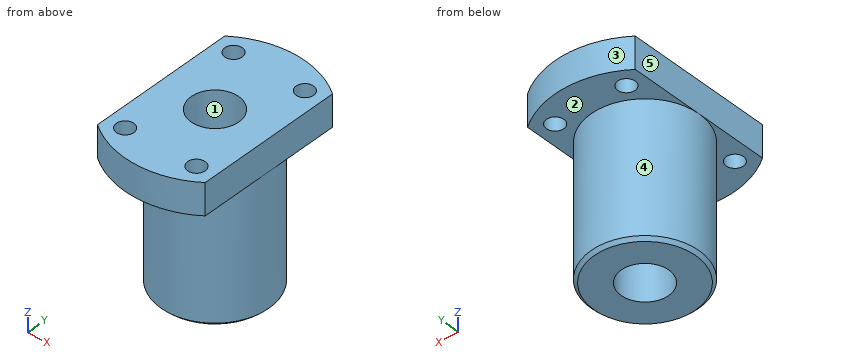
```python
from build123d import *

# Parameters (mm, degrees)
SKETCH_1_R          = 28.5
EXTRUDE_1_DEPTH     = 10
SKETCH_2_W          = 42.780685773
SKETCH_2_H          = 76.581039372
CUT_EXTRUDE_1_DEPTH = 42.527099586
SKETCH_3_R          = 17
EXTRUDE_2_DEPTH     = 42
SKETCH_4_R          = 2.75
CUT_EXTRUDE_2_DEPTH = 42
SKETCH_5_R          = 7.5
CUT_EXTRUDE_3_DEPTH = 62.686708455
CHAMFER_1_SIZE      = 1


with BuildPart() as part:
    # 草图1 → 凸台-拉伸1 (new body)
    with BuildSketch(Plane.XY):
        Circle(SKETCH_1_R)
    extrude(amount=EXTRUDE_1_DEPTH)

    # 草图2 → 切除-拉伸1 (cut, through all)
    with BuildSketch(Plane.XY.offset(10)):
        with Locations((-38.390342887, -1.01716671)):
            Rectangle(SKETCH_2_W, SKETCH_2_H)
        with Locations((38.390342887, -1.01716671)):
            Rectangle(SKETCH_2_W, SKETCH_2_H)
    extrude(amount=-CUT_EXTRUDE_1_DEPTH, mode=Mode.SUBTRACT)

    # 草图3 → 凸台-拉伸2 (add)
    with BuildSketch(Plane(origin=(0, 0, 0), x_dir=(-1, 0, 0), z_dir=(0, 0, -1))):
        Circle(SKETCH_3_R)
    extrude(amount=EXTRUDE_2_DEPTH)

    # 草图4 → 切除-拉伸2 (cut)
    with BuildSketch(Plane(origin=(0, 0, 0), x_dir=(-1, 0, 0), z_dir=(0, 0, -1))):
        with Locations((-11.25, 19.485571585)):
            Circle(SKETCH_4_R)
        with Locations((11.25, 19.485571585)):
            Circle(SKETCH_4_R)
        with Locations((11.25, -19.485571585)):
            Circle(SKETCH_4_R)
        with Locations((-11.25, -19.485571585)):
            Circle(SKETCH_4_R)
    extrude(amount=-CUT_EXTRUDE_2_DEPTH, mode=Mode.SUBTRACT)

    # 草图5 → 切除-拉伸3 (cut, through all)
    with BuildSketch(Plane.XY.offset(10)):
        Circle(SKETCH_5_R)
    extrude(amount=-CUT_EXTRUDE_3_DEPTH, mode=Mode.SUBTRACT)

    # 倒角1
    chamfer_1_edges = [part.edges().sort_by_distance(p)[0] for p in [
        (17, 0, -42),
    ]]
    chamfer(chamfer_1_edges, length=CHAMFER_1_SIZE)


solid = part.part
```
Geometry check sheet. Reference: the model listing, model coordinates, mm. Face numbers are marked on the shaded views. A direction names the side the tool comes from. Give positions to 0.01 mm unless a question says otherwise; leave off trailing zeros. Loops run counter-clockwise (first coordinate to the right, second up) from the corner with the lowest first, then second, coordinate; pieces in that order, holes last. Notation, with made-up numbers: M 29.5,-23 L 86.5,-23 A18 ccw 86.5,11 Z; hole C 30.25,60.5 d1. An arc over 180 degrees is marked long. Write item = value, one per line. Start each with the question number.
1. Draft check along X on the marked faces 1, 2 and 3. Enter one of: +X half, -X half, draft (parallel to the pull), parting line (faces both ways), or undercut.
2. Thickness scan on probe 1 along Y at (x, z) = (11.25, 6.25); probe 2 along Y at (x, z) = (1, -34.5); probe 3 along X at (y, z) = (6.5, -13.5). Record the ranges inside material, lowest first.
3. Go/stop test with flat-tipped pins: P1, Ø5, axis at y = 11.5, z = -19.5, coming from the +X side; P2, Ø10, axis at y = 15, z = -1, coming from the -X side; P3, Ø1.5, axis at x = 2, z = -33, coming from the -Y side; P4, Ø8, axis at y = 19, z = -26, coming from the -X side. Record where each tip stops, or that it passes through.
4. Section check A-A, the plane x = 0. Enter the section's corners in (y, z), plus the area to 3 significant figures.
5. Section check B-B, the plane x = -9.5. Give the number of separate pieces and of enclosed holes in the cut face, plus the area to 3 significant figures.
6. Tool access check on the marked faces 4 and 5. Record the directions out of +Z, -Z, +X, -X, +Y, -Y that give a thin tool (end or side, any length) a straight path to the whole face; none if there is none.
Values follow:
q1.face_1 = undercut
q1.face_2 = draft
q1.face_3 = parting line
q2.probe_1 = -26.19 to -22.24, -16.74 to 16.74, 22.24 to 26.19
q2.probe_2 = -16.97 to -7.43, 7.43 to 16.97
q2.probe_3 = -15.71 to -3.74, 3.74 to 15.71
q3.P1 = 14.42
q3.P2 = -17
q3.P3 = -16.95
q3.P4 = -8
q4.outline = M -28.5,0 L -17,0 L -17,-41 L -16,-42 L -7.5,-42 L -7.5,10 L -28.5,10 Z; M 7.5,-42 L 16,-42 L 17,-41 L 17,0 L 28.5,0 L 28.5,10 L 7.5,10 Z
q4.area = 1,220 mm^2
q5.separate_pieces = 3
q5.enclosed_holes = 0
q5.area = 1,640 mm^2
q6.face_4 = -Z
q6.face_5 = +Z, -Z, -X, +Y, -Y
